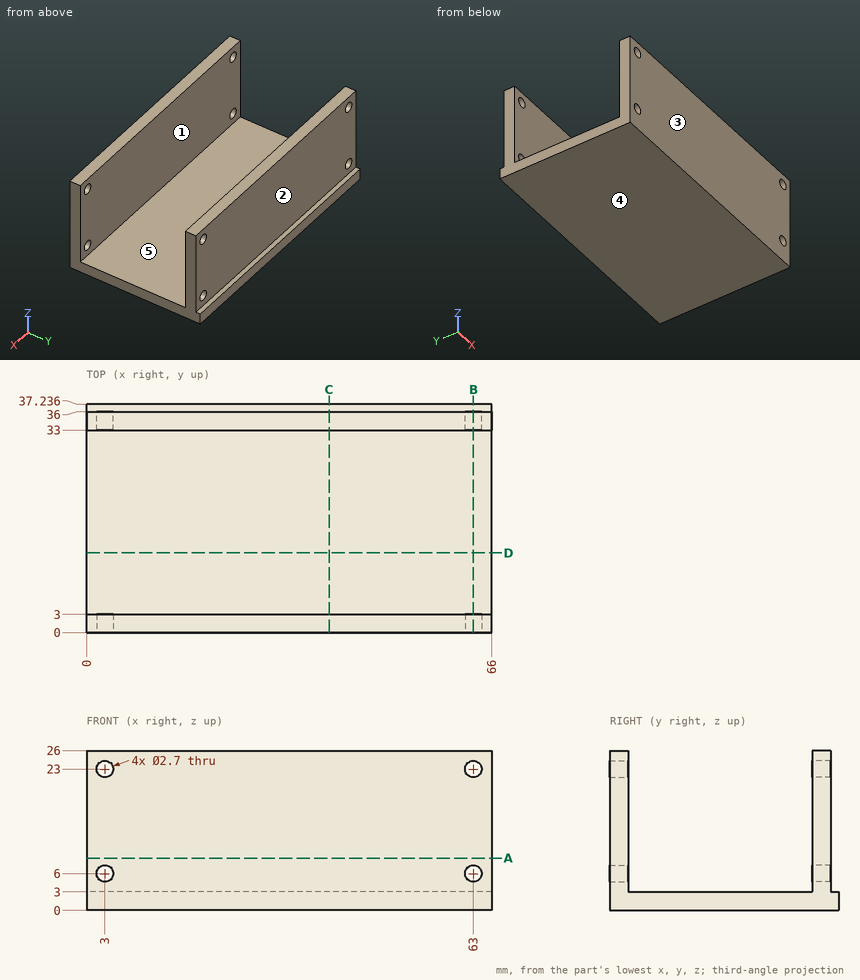
The drawing under review shows one solid part. Ordinate dimensions are in mm from its lowest x, y, z. A direction names the side the tool comes from. Coordinates: 2 decimals unless noted, no trailing zeros. Write each loop counter-clockwise with the first axis right and the second up, starting at its lowest first coordinate (ties: lowest second). Pieces come first, ordered by that corner, then holes. Notation, with made-up numbers: (-11, 12.5) - (22, 12.5) arc R18 cw to (22, 18.5) - close; hole circle Ø4 at (52, -20). An arc over 180 degrees is marked (long way). Put each result on its own line as item: value.
1. Add section A-A, the plane z = 8.5. Give the boundary of the cut face in (x, y).
Values found:
outline: (0, 0) - (66, 0) - (66, 3) - (0, 3) - close; (0, 33) - (66, 33) - (66, 36) - (0, 36) - close
2. Add section B-B, the plane x = 63. Give the boundary of the cut face in (y, z), then the cut area to 3 significant figures.
Values found:
outline: (0, 0) - (37.24, 0) - (37.24, 3) - (36, 3) - (36, 4.65) - (33, 4.65) - (33, 3) - (3, 3) - (3, 4.65) - (0, 4.65) - close; (0, 7.35) - (3, 7.35) - (3, 21.65) - (0, 21.65) - close; (0, 24.35) - (3, 24.35) - (3, 26) - (0, 26) - close; (33, 7.35) - (36, 7.35) - (36, 21.65) - (33, 21.65) - close; (33, 24.35) - (36, 24.35) - (36, 26) - (33, 26) - close
area: 217 mm²
3. Mouldability with a two-part tool opening along Y and no side actions: class the marked faces 3, 4 and 5 as released by +Y, released by -Y, zero draft, split by the parting line, or undercut.
Values found:
face 3: released by -Y
face 4: zero draft
face 5: undercut
4. For pin 1 (5 mm diameter, centred on y = 28.5, z = 10.5, fed in from -X); pin 2 (11.5 mm diameter, centred on x = 33, z = 9.5, fed in from +Y); pin 3 (8 mm diameter, centred on x = 46.5, y = 14.5, fed in from +Z); pin 4 (3 mm diameter, centred on x = 17.5, z = 17.5, fed in from -Y), all flat-tipped, find the tip position at first contact; note any pin that passes through.
Values found:
pin 1: through
pin 2: y = 36
pin 3: z = 3
pin 4: y = 0
5. Wall thickness on probe 1 along Z at (x, y) = (63, 1); probe 2 along X at (y, z) = (35.1, 6); probe 3 along Y at (x, z) = (54.5, 9.5): over which ranges is each line inside the solid? List them lowest first.
Values found:
probe 1: 0 to 4.65, 7.35 to 21.65, 24.35 to 26
probe 2: 0 to 1.65, 4.35 to 61.65, 64.35 to 66
probe 3: 0 to 3, 33 to 36
6. Machinability: for the marked faces 1 and 2, which of the approach directions +Z, -Z, +X, -X, +Y, -Y give a long, thin tool a straight path to every point of the face, cutting with its end or side? Answer none if there is none.
Values found:
face 1: +Z, +X, -X
face 2: +Z, +X, -X, +Y
7. Add section D-D, the plane y = 13. Give the boundary of the cut face in (x, z).
Values found:
outline: (0, 0) - (66, 0) - (66, 3) - (0, 3) - close
8. Add section C-C, the plane x = 39.5. Give the boundary of the cut face in (y, z).
Values found:
outline: (0, 0) - (37.24, 0) - (37.24, 3) - (36, 3) - (36, 26) - (33, 26) - (33, 3) - (3, 3) - (3, 26) - (0, 26) - close
